Autodesk Inventor part; units mm, degrees
ref_plane "YZ Plane" through (0, 0, 0) normal (1, 0, 0) x (0, 1, 0)
ref_plane "XZ Plane" through (0, 0, 0) normal (0, 1, 0) x (-1, 0, 0)
ref_plane "XY Plane" through (0, 0, 0) normal (0, 0, 1) x (1, 0, 0)
sketch "Sketch9" plane through (0, 0, 0) normal (1, 0, 0) x (0, 1, 0)
  arc A0 (-11.2991, -17.7011) -> (-11.2991, 17.7011) centre (0, 0) ccw
  arc A1 (-9.6991, -20.4129) -> (-9.6991, 20.4129) centre (0, 0) ccw
  line L0 (-9.6991, 45) -> (-11.2991, 45)
  line L1 (-11.2991, 45) -> (-11.2991, 17.7011)
  line L2 (-9.6991, 0) -> (-16.1126, 0) construction
  line L3 (-9.6991, -45) -> (-11.2991, -45)
  line L4 (-11.2991, -45) -> (-11.2991, -17.7011)
  line L5 (-9.6991, 45) -> (-9.6991, 18.626)
  line L6 (-9.6991, -18.626) -> (-9.6991, -45)
  dimension "d36" = 42
  dimension "d37" = 45.2
  dimension "d38" = 90
  dimension "d39" = 45
  dimension "d40" = 1.6
extrude "Extrusion5" add sketch "Sketch9" along normal blind 8
sketch "Sketch10" plane through (0, -9.6991, 45) normal (0, 1, 0) x (1, 0, 0)
  circle A0 centre (4, 10) radius 2.9
  circle A1 centre (4, 80) radius 2.9
  line L0 (0, 0) -> (8, 0)
  line L1 (0, 90) -> (8, 90)
  line L2 (8, 90) -> (8, 65.4129)
  line L3 (0, 24.5871) -> (0, 0)
  point P0 (0, 45)
  dimension "d43" = 5.8
  dimension "d44" = 5.8
  dimension "d45" = 10
  dimension "d46" = 10
  dimension "d47" = 4
  dimension "d48" = 4
extrude "Extrusion6" cut sketch "Sketch10" against normal through all
Could you check a few things on this model? Use its own coordinates, in mm. A direction names the side the tool comes from. Give positions to 0.01 mm unless a question says otherwise; leave off trailing zeros. Loops run counter-clockwise (first coordinate to the right, second up) from the corner with the lowest first, then second, coordinate; pieces in that order, holes last. Notation, with made-up numbers: M 39,89 L 49,89 A32 cw 49,120 Z; hole C 35.25,9 d6. An arc over 180 degrees is marked long. Answer as a JSON object with one key per item and string values.
Q1. Suppose I cut it at D-D, the plane z = -29.5. List the corners of the cut face in (x, y) for me.
Values found:
{"outline": "M 0,-11.3 L 8,-11.3 L 8,-9.7 L 0,-9.7 Z"}
Q2. Suppose I cut it at B-B, the plane x = 4. List the corners of the cut face in (y, z) for me.
Values found:
{"outline": "M -11.3,-45 L -9.7,-45 L -9.7,-37.9 L -11.3,-37.9 Z; M -11.3,-32.1 L -9.7,-32.1 L -9.7,-20.41 A22.6 ccw long -9.7,20.41 L -9.7,32.1 L -11.3,32.1 L -11.3,17.7 A21 cw long -11.3,-17.7 Z; M -11.3,37.9 L -9.7,37.9 L -9.7,45 L -11.3,45 Z"}
Q3. Suppose I cut it at A-A, the plane z = 35. List the corners of the cut face in (x, y) for me.
Values found:
{"outline": "M 0,-11.3 L 1.1,-11.3 L 1.1,-9.7 L 0,-9.7 Z; M 6.9,-11.3 L 8,-11.3 L 8,-9.7 L 6.9,-9.7 Z"}
Q4. Suppose I cut it at C-C, the plane y = 2.5. List the corners of the cut face in (x, z) for me.
Values found:
{"outline": "M 0,-22.46 L 8,-22.46 L 8,-20.85 L 0,-20.85 Z; M 0,20.85 L 8,20.85 L 8,22.46 L 0,22.46 Z"}
Q5. If I drill on probe 1 along Z at (x, y) = (3.25, 0); probe 2 along X at (y, z) = (-10, 35); probe 3 along Z at (x, y) = (4, -10.1), over which ranges is the centre line in solid material (lowest first)? Write a range as [from, to].
Values found:
{"probe 1": "z = [-22.6, -21], [21, 22.6]", "probe 2": "x = [0, 1.1], [6.9, 8]", "probe 3": "z = [-45, -37.9], [-32.1, -18.41], [18.41, 32.1], [37.9, 45]"}
Q6. For faces 4 (the flat face through (4, -9.699, 30)), 5 (the flat face through (2.2, -9.699, -32.5)), 6 (the cylindrical face through (3.37, -10.49, -32.17)), which set-ups out of +Z, -Z, +X, -X, +Y, -Y let a thin tool reach every point of the face, with its end or its side?
Values found:
{"face 4": "+Z, +X, -X", "face 5": "-Z, +X, -X", "face 6": "+Y, -Y"}
Q7. For P1, Ø2, axis at x = 1, z = 20.5, coming from the +Y side; P2, Ø12, axis at y = 5, z = 23.5, coming from the +X side; P3, Ø1, axis at x = 5.5, z = -1.5, coming from the -Y side; P4, Ø2.5, axis at x = 2.5, z = -38.5, coming from the +Y side, each with a flat end and sliding along its axis, tell me the tip position at first contact or that it passes through.
Values found:
{"P1": "stops at y = 11.42", "P2": "stops at x = 8", "P3": "stops at y = 20.9", "P4": "stops at y = -9.7"}
Q8. If we mould it in two halves opening along Z, with no side actions, what happens to faces 1 (the flat face through (4, -10, -45)), 2 (the cylindrical face through (3.94, 20.99, 0.63)), 3 (the flat face through (8, 13, 17))? For each: pulls with the +Z half, pulls with the -Z half, needs draft (parallel to the pull), parting line crosses it, or undercut.
Values found:
{"face 1": "pulls with the -Z half", "face 2": "undercut", "face 3": "needs draft"}
